Autodesk Inventor part; units mm, degrees
ref_plane "YZ Plane" through (0, 0, 0) normal (1, 0, 0) x (0, 1, 0)
ref_plane "XZ Plane" through (0, 0, 0) normal (0, 1, 0) x (-1, 0, 0)
ref_plane "XY Plane" through (0, 0, 0) normal (0, 0, 1) x (1, 0, 0)
sketch "Эскиз1" plane through (0, 0, 0) normal (0, 1, 0) x (-1, 0, 0)
  line L0 (-4.3301, -7.5) -> (-8.6603, 0)
  line L1 (-8.6603, 0) -> (-4.3301, 7.5)
  line L2 (-4.3301, 7.5) -> (4.3301, 7.5)
  line L3 (4.3301, 7.5) -> (8.6603, 0)
  line L4 (8.6603, 0) -> (4.3301, -7.5)
  line L5 (4.3301, -7.5) -> (-4.3301, -7.5)
  circle A0 centre (0, 0) radius 5.6
  dimension "d0" = 15
  dimension "d1" = 11.2
extrude "Выдавливание1" add sketch "Эскиз1" along normal blind 2.8
chamfer "Фаска1" distance 1 angle 30 6 edges at (0, 2.8, 7.5) (6.4952, 2.8, 3.75) (6.4952, 2.8, -3.75) (0, 2.8, -7.5) (-6.4952, 2.8, -3.75) (-6.4952, 2.8, 3.75) measured on face at (0.225, 2.8, 6.8531)
chamfer "Фаска2" distance 1 angle 30 6 edges at (-6.4952, 0, 3.75) (0, 0, 7.5) (6.4952, 0, 3.75) (6.4952, 0, -3.75) (0, 0, -7.5) (-6.4952, 0, -3.75) measured on face at (0.225, 0, 6.8531)
thread "Резьба1"
chamfer "Фаска3" distance 0.3 angle 45 2 edges at (5.6, 2.8, 0) (5.6, 0, 0)
properties part number "гайка" material "Сталь, нержавеющая, полированная"
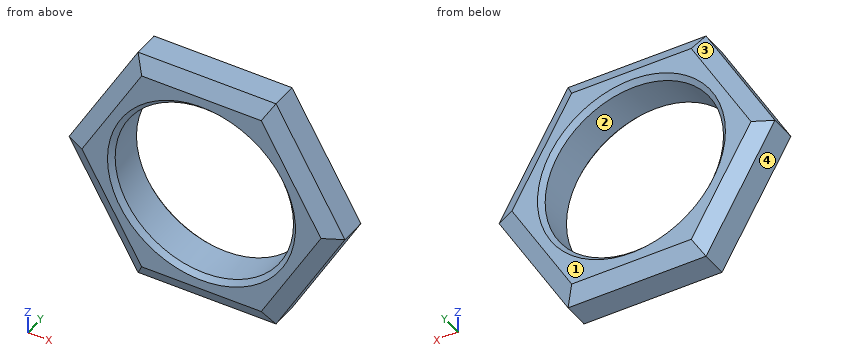
Build history of the part. All positions in model axes, mm. Face numbers are marked on the shaded views. Coordinates: 2 decimals unless noted, no trailing zeros. Order: outer loops, then holes, each group sorted by start corner. A loop starts at its lowest first (then second) coordinate and runs counter-clockwise, first axis right, second up. Notation, with made-up numbers: (-22, 44.5) - (34, 44.5) arc R20 ccw to (34, 51.5) - close; hole circle Ø7 at (-14, 2). An arc over 180 degrees is marked (long way). Put each result on its own line as item: value.
1. Saw through at B-B (x = 0). Write the cut outline in (y, z).
Answer sheet:
outline: (0, -6.5) - (0.58, -7.5) - (2.22, -7.5) - (2.8, -6.5) - (2.8, -5.9) - (2.5, -5.6) - (0.3, -5.6) - (0, -5.9) - close; (0, 5.9) - (0.3, 5.6) - (2.5, 5.6) - (2.8, 5.9) - (2.8, 6.5) - (2.22, 7.5) - (0.58, 7.5) - (0, 6.5) - close
2. Saw through at C-C (x = 7). Write the cut outline in (y, z).
Answer sheet:
outline: (0, -0.88) - (0.58, -2.88) - (2.22, -2.88) - (2.8, -0.88) - (2.8, 0.88) - (2.22, 2.88) - (0.58, 2.88) - (0, 0.88) - close
3. Probe line 1 along Z through (x, y) = (0, 1.05); line 2 along X through (y, z) = (1.35, -3.25); line 3 along X through (y, z) = (1.35, 4.5). List the from-to ranges inside material, lowest first. Write a range as [from, to].
Answer sheet:
line 1: z = [-7.5, -5.6], [5.6, 7.5]
line 2: x = [-6.78, -4.56], [4.56, 6.78]
line 3: x = [-6.06, -3.33], [3.33, 6.06]
4. Saw through at A-A (y = 1.3). Write the cut outline in (x, z).
Answer sheet:
outline: (-8.66, 0) - (-4.33, -7.5) - (4.33, -7.5) - (8.66, 0) - (4.33, 7.5) - (-4.33, 7.5) - close; hole circle Ø11.2 at (0, 0)
5. Pull direction Z, two halves, no side cores. Call the marked faces 1, 2, 3 and 4: pulls with the +Z half, pulls with the -Z half, needs draft (parallel to the pull), parting line crosses it, or undercut.
Answer sheet:
face 1: needs draft
face 2: undercut
face 3: pulls with the +Z half
face 4: pulls with the -Z half
